The model under review builds one solid part; all positions refer to its coordinate system, in mm. A direction names the side the tool comes from. Round coordinates to 2 decimals unless told otherwise and drop trailing zeros. Order: outer loops, then holes, each group sorted by start corner. A loop starts at its lowest first (then second) coordinate and runs counter-clockwise, first axis right, second up. Notation, with made-up numbers: (49.5, 42) -> (87.5, 42) arc R14 cw to (87.5, 53) -> close; hole circle Ø10 at (-14.75, -25). An arc over 180 degrees is marked (long way). Return JSON: item names as keys, results as strings. Group by question number.
from build123d import *

# Parameters (mm, degrees)
SKETCH1_W            = 25.4
SKETCH1_H            = 25.4
BOSS_EXTRUDE1_DEPTH  = 56.75
SKETCH2_W            = 23.8125
SKETCH2_H            = 23.8125
CUT_EXTRUDE1_DEPTH   = 115.912270885
FILLET1_R            = 0.508
M3_CLEARANCE_HOLE1_D = 3.4
M3_CLEARANCE_HOLE2_D = 3.4
M3_CLEARANCE_HOLE3_D = 3.4
M3_CLEARANCE_HOLE4_D = 3.4
FILLET2_R            = 1.5
CUT_EXTRUDE2_REACH   = 65.459
SKETCH11_W           = 16.9
SKETCH11_H           = 6.499999954
SKETCH11_H_2         = 7
CUT_EXTRUDE3_REACH   = 65.459
SKETCH12_W           = 16.9
SKETCH12_H           = 6.5
SKETCH12_H_2         = 7
FILLET3_R            = 3.81
CUT_EXTRUDE4_REACH   = 65.459
SKETCH13_W           = 15.4
SKETCH13_H           = 87.3
CUT_EXTRUDE5_REACH   = 65.459
SKETCH14_W           = 15.4
SKETCH14_H           = 87.3
CHAMFER2_SIZE        = 6.35
FILLET5_R            = 3.81
SKETCH15_W           = 12.31
SKETCH15_H           = 12.31
CUT_EXTRUDE6_DEPTH   = 6.5
SKETCH17_W           = 12.31
SKETCH17_H           = 12.31
CUT_EXTRUDE8_DEPTH   = 7
BOSS_EXTRUDE2_START  = -1.5875
BOSS_EXTRUDE2_DEPTH  = 1.5875
BOSS_EXTRUDE3_START  = -1.5875
BOSS_EXTRUDE3_DEPTH  = 1.5875
SKETCH22_W           = 10.5875
SKETCH22_H           = 10.5875
CUT_EXTRUDE9_DEPTH   = 2
FILLET6_R            = 0.5
FILLET6_OF_MIRROR1_R = 0.5


with BuildPart() as part:
    # Sketch1 → Boss-Extrude1 (new, symmetric)
    with BuildSketch(Plane(origin=(0, 0, 0), x_dir=(1, 0, 0), z_dir=(0, 1, 0))):
        Rectangle(SKETCH1_W, SKETCH1_H)
    extrude(amount=BOSS_EXTRUDE1_DEPTH, both=True)

    # Sketch2 → Cut-Extrude1 (cut, through all)
    with BuildSketch(Plane(origin=(0, 56.75, 0), x_dir=(1, 0, 0), z_dir=(0, 1, 0))):
        with Locations((0.79375, 0.79375)):
            Rectangle(SKETCH2_W, SKETCH2_H)
    extrude(amount=-CUT_EXTRUDE1_DEPTH, mode=Mode.SUBTRACT)

    # Fillet1
    fillet1_edges = [part.edges().sort_by_distance(p)[0] for p in [
        (-11.1125, 0, 11.1125),
    ]]
    fillet(fillet1_edges, radius=FILLET1_R)

    # M3 Clearance Hole1 (through all)
    with Locations(Plane.XY.offset(12.7)):
        with Locations((6.35, 47.075)):
            Hole(M3_CLEARANCE_HOLE1_D / 2)

    # M3 Clearance Hole2 (through all)
    with Locations(Plane.ZY.offset(12.7)):
        with Locations((-6.35, 47.075)):
            Hole(M3_CLEARANCE_HOLE2_D / 2)

    # M3 Clearance Hole3 (through all)
    with Locations(Plane.XY.offset(12.7)):
        with Locations((6.35, -46.575)):
            Hole(M3_CLEARANCE_HOLE3_D / 2)

    # M3 Clearance Hole4 (through all)
    with Locations(Plane.ZY.offset(12.7)):
        with Locations((-6.35, -46.575)):
            Hole(M3_CLEARANCE_HOLE4_D / 2)

    # Fillet2
    fillet2_edges = [part.edges().sort_by_distance(p)[0] for p in [
        (-12.7, 0, 12.7),
    ]]
    fillet(fillet2_edges, radius=FILLET2_R)

    # Sketch11 → Cut-Extrude2 (cut, up to next)
    with BuildSketch(Plane.ZY.offset(12.7), mode=Mode.PRIVATE) as cut_extrude2_sk1:
        with Locations((-4.25, 53.500000023)):
            Rectangle(SKETCH11_W, SKETCH11_H)
    cut_extrude2_tool1 = extrude(cut_extrude2_sk1.sketch, amount=-CUT_EXTRUDE2_REACH, mode=Mode.PRIVATE) & part.part
    # Sketch11 → Cut-Extrude2 (cut, up to next)
    with BuildSketch(Plane.ZY.offset(12.7), mode=Mode.PRIVATE) as cut_extrude2_sk2:
        with Locations((-4.25, -53.25)):
            Rectangle(SKETCH11_W, SKETCH11_H_2)
    cut_extrude2_tool2 = extrude(cut_extrude2_sk2.sketch, amount=-CUT_EXTRUDE2_REACH, mode=Mode.PRIVATE) & part.part
    add(cut_extrude2_tool1.solids().sort_by_distance((-12.7, 53.5, -4.25))[0], mode=Mode.SUBTRACT)
    add(cut_extrude2_tool2.solids().sort_by_distance((-12.7, -53.25, -4.25))[0], mode=Mode.SUBTRACT)

    # Sketch12 → Cut-Extrude3 (cut, up to next)
    with BuildSketch(Plane.XY.offset(12.7), mode=Mode.PRIVATE) as cut_extrude3_sk1:
        with Locations((4.25, 53.5)):
            Rectangle(SKETCH12_W, SKETCH12_H)
    cut_extrude3_tool1 = extrude(cut_extrude3_sk1.sketch, amount=-CUT_EXTRUDE3_REACH, mode=Mode.PRIVATE) & part.part
    # Sketch12 → Cut-Extrude3 (cut, up to next)
    with BuildSketch(Plane.XY.offset(12.7), mode=Mode.PRIVATE) as cut_extrude3_sk2:
        with Locations((4.25, -53.25)):
            Rectangle(SKETCH12_W, SKETCH12_H_2)
    cut_extrude3_tool2 = extrude(cut_extrude3_sk2.sketch, amount=-CUT_EXTRUDE3_REACH, mode=Mode.PRIVATE) & part.part
    add(cut_extrude3_tool1.solids().sort_by_distance((4.25, 53.5, 12.7))[0], mode=Mode.SUBTRACT)
    add(cut_extrude3_tool2.solids().sort_by_distance((4.25, -53.25, 12.7))[0], mode=Mode.SUBTRACT)

    # Fillet3
    fillet3_edges = [part.edges().sort_by_distance(p)[0] for p in [
        (-4.2, 50.25, 11.90625),
        (-4.2, -49.75, 11.90625),
        (-11.90625, 50.250000046, 4.2),
        (-11.90625, -49.75, 4.2),
    ]]
    fillet(fillet3_edges, radius=FILLET3_R)

    # Sketch13 → Cut-Extrude4 (cut, up to next)
    with BuildSketch(Plane.ZY.offset(12.7), mode=Mode.PRIVATE) as cut_extrude4_sk1:
        with Locations((-5, 0.25)):
            Rectangle(SKETCH13_W, SKETCH13_H)
    cut_extrude4_tool1 = extrude(cut_extrude4_sk1.sketch, amount=-CUT_EXTRUDE4_REACH, mode=Mode.PRIVATE) & part.part
    add(cut_extrude4_tool1.solids().sort_by_distance((-12.7, 0.25, -5))[0], mode=Mode.SUBTRACT)

    # Sketch14 → Cut-Extrude5 (cut, up to next)
    with BuildSketch(Plane.XY.offset(12.7), mode=Mode.PRIVATE) as cut_extrude5_sk1:
        with Locations((5, 0.25)):
            Rectangle(SKETCH14_W, SKETCH14_H)
    cut_extrude5_tool1 = extrude(cut_extrude5_sk1.sketch, amount=-CUT_EXTRUDE5_REACH, mode=Mode.PRIVATE) & part.part
    add(cut_extrude5_tool1.solids().sort_by_distance((5, 0.25, 12.7))[0], mode=Mode.SUBTRACT)

    # Chamfer2
    chamfer2_edges = [part.edges().sort_by_distance(p)[0] for p in [
        (-11.90625, 43.9, 2.7),
        (-11.90625, -43.4, 2.7),
        (-2.7, -43.4, 11.90625),
        (-2.7, 43.9, 11.90625),
    ]]
    chamfer(chamfer2_edges, length=CHAMFER2_SIZE)

    # Fillet5
    fillet5_edges = [part.edges().sort_by_distance(p)[0] for p in [
        (-11.90625, 43.9, -3.65),
        (-11.90625, -37.05, 2.7),
        (-11.90625, 37.55, 2.7),
        (-2.7, -37.05, 11.90625),
        (-2.7, 37.55, 11.90625),
        (3.65, 43.9, 11.90625),
        (3.65, -43.4, 11.90625),
        (-11.90625, -43.4, -3.65),
    ]]
    fillet(fillet5_edges, radius=FILLET5_R)

    # Sketch15 → Cut-Extrude6 (cut)
    with BuildSketch(Plane(origin=(0, 56.75, 0), x_dir=(1, 0, 0), z_dir=(0, 1, 0))):
        with Locations((-6.545, -6.545)):
            Rectangle(SKETCH15_W, SKETCH15_H)
    extrude(amount=-CUT_EXTRUDE6_DEPTH, mode=Mode.SUBTRACT)

    # Sketch17 → Cut-Extrude8 (cut)
    with BuildSketch(Plane.XZ.offset(56.75)):
        with Locations((-6.545, 6.545)):
            Rectangle(SKETCH17_W, SKETCH17_H)
    extrude(amount=-CUT_EXTRUDE8_DEPTH, mode=Mode.SUBTRACT)

    # Sketch20 → Boss-Extrude2 (add)
    with BuildSketch(Plane.ZY.offset(12.7).offset(BOSS_EXTRUDE2_START)):
        with BuildLine():
            Line((-12.7, 43.9), (-12.7, -43.4))
            Line((-12.7, -43.4), (-5.228153673, -43.4))
            ThreePointArc((-5.228153673, -43.4), (-3.770129795, -43.109981019), (-2.534076836, -42.284076836))
            Line((-2.534076836, -42.284076836), (1.584076836, -38.165923164))
            ThreePointArc((1.584076836, -38.165923164), (2.409981019, -36.929870205), (2.7, -35.471846327))
            Line((2.7, -35.471846327), (2.7, 35.971846327))
            ThreePointArc((2.7, 35.971846327), (2.409981019, 37.429870205), (1.584076836, 38.665923164))
            Line((1.584076836, 38.665923164), (-2.534076836, 42.784076836))
            ThreePointArc((-2.534076836, 42.784076836), (-3.770129795, 43.609981019), (-5.228153673, 43.9))
            Line((-5.228153673, 43.9), (-12.7, 43.9))
        make_face()
    extrude(amount=BOSS_EXTRUDE2_DEPTH)

    # Sketch21 → Boss-Extrude3 (add)
    with BuildSketch(Plane.XY.offset(12.7).offset(BOSS_EXTRUDE3_START)):
        with BuildLine():
            Line((12.7, 43.9), (12.7, -43.4))
            Line((12.7, -43.4), (5.228153673, -43.4))
            ThreePointArc((5.228153673, -43.4), (3.770129795, -43.109981019), (2.534076836, -42.284076836))
            Line((2.534076836, -42.284076836), (-1.584076836, -38.165923164))
            ThreePointArc((-1.584076836, -38.165923164), (-2.409981019, -36.929870205), (-2.7, -35.471846327))
            Line((-2.7, -35.471846327), (-2.7, 35.971846327))
            ThreePointArc((-2.7, 35.971846327), (-2.409981019, 37.429870205), (-1.584076836, 38.665923164))
            Line((-1.584076836, 38.665923164), (2.534076836, 42.784076836))
            ThreePointArc((2.534076836, 42.784076836), (3.770129795, 43.609981019), (5.228153673, 43.9))
            Line((5.228153673, 43.9), (12.7, 43.9))
        make_face()
    extrude(amount=BOSS_EXTRUDE3_DEPTH)

    # Sketch22 → Cut-Extrude9 (cut)
    with BuildSketch(Plane(origin=(0, 50.250000046, 0), x_dir=(1, 0, 0), z_dir=(0, 1, 0))):
        with Locations((-7.40625, -7.40625)):
            Rectangle(SKETCH22_W, SKETCH22_H)
    cut_extrude9 = extrude(amount=-CUT_EXTRUDE9_DEPTH, mode=Mode.SUBTRACT)

    # Fillet6
    fillet6_edges = [part.edges().sort_by_distance(p)[0] for p in [
        (-11.90625, 48.250000046, 2.1125),
        (-2.1125, 48.250000046, 11.90625),
    ]]
    fillet(fillet6_edges, radius=FILLET6_R)

    # Mirror1: Cut-Extrude9 across plane
    add(cut_extrude9.mirror(Plane.ZX.offset(0.250000023)), mode=Mode.SUBTRACT)

    # Fillet6 of Mirror1
    fillet6_of_mirror1_edges = [part.edges().sort_by_distance(p)[0] for p in [
        (-11.90625, -47.75, 2.1125),
        (-2.1125, -47.75, 11.90625),
    ]]
    fillet(fillet6_of_mirror1_edges, radius=FILLET6_OF_MIRROR1_R)


solid = part.part
Item 1: Consider section C-C on y = -31.5. State the section outline as (x, z) points, plus the area to 3 significant figures.
Item 2: The part is to be moulded in two halves that separate along Y. For faces 1 (the face through (1, 1, 11.112)), 2 (the face through (-11.4, 48.25, 9.5)), 3 (the face through (-11.895, 45.415, -5.981)), say which applies: +Y half, -Y half, draft (parallel to the pull), parting line (faces both ways), or undercut.
Item 3: Consider section D-D on x = -8.5. State the section outline as (y, z) points, plus the area to 3 significant figures.
Item 4: Consider section A-A on x = 6.35. Give the number of separate pieces and of enclosed holes in the cut face, plus the area to 3 significant figures.
Item 5: Wall thickness on line 1 along Y through (x, z) = (-11.45, -6.35) (3 decimals); line 2 along Z through (x, y) = (2, -27); line 3 along X through (y, z) = (-41, 4.5): over which ranges is each line inside the solid? List them lowest first.
Item 6: For faces 4 (the face through (-11.4, -47.75, 9.5)), 5 (the face through (-11.895, -45.426, -5.097)), 6 (the face through (-11.112, 1, -1)), list the 3-axis set-ups (+Z, -Z, +X, -X, +Y, -Y) from which the entire face can be reached by the end or side of a thin tool; tool diameter is ignored.
Item 7: Insertion check: pin 1 Ø4.5 at (x, y) = (6.35, 47.075) entering from -Z; pin 2 Ø0.8 at (y, z) = (-49, 12) entering from -X; pin 3 Ø1.6 at (x, y) = (-12.5, -49) entering from +Z (3 decimals). Each pin has a flat end and moves straight along its axis. Give the tip position at first contact, or say it passes through.
Values:
{
 "1": {"outline": "(-12.7, -12.7) -> (-11.11, -12.7) -> (-11.11, 10.6) arc R0.51 cw to (-10.6, 11.11) -> (12.7, 11.11) -> (12.7, 12.7) -> (-11.2, 12.7) arc R1.5 ccw to (-12.7, 11.2) -> close", "area": "77.7 mm^2"},
 "2": {"face 1": "draft", "face 2": "+Y half", "face 3": "undercut"},
 "3": {"outline": "(-47.75, 11.11) -> (48.25, 11.11) -> (48.25, 12.7) -> (-47.75, 12.7) -> close", "area": "152 mm^2"},
 "4": {"separate pieces": "3", "enclosed holes": "0", "area": "148 mm^2"},
 "5": {"line 1": "-49.75 to -48.275, -44.875 to 45.375, 48.775 to 50.25", "line 2": "11.11 to 12.7", "line 3": "-12.7 to -11.11"},
 "6": {"face 4": "+Z, -X, -Y", "face 5": "+X, -X", "face 6": "-Z, +X, +Y, -Y"},
 "7": {"pin 1": "z = 11.11", "pin 2": "x = -2.11", "pin 3": "z = 2.115"}
}
